from build123d import *

# Parameters (mm, degrees)
SKETCH1_W               = 110
SKETCH1_H               = 31.4
BOSS_EXTRUDE1_DEPTH     = 6
SKETCH2_R               = 2.54
SKETCH2_R_2             = 5
SKETCH2_R_3             = 2.5
CUT_EXTRUDE1_DEPTH      = 1
CUT_EXTRUDE1_DEPTH_BACK = 7


with BuildPart() as part:
    # Sketch1 → Boss-Extrude1 (new body)
    with BuildSketch(Plane(origin=(0, 0, 0), x_dir=(1, 0, 0), z_dir=(0, 1, 0))):
        Rectangle(SKETCH1_W, SKETCH1_H)
    extrude(amount=BOSS_EXTRUDE1_DEPTH)

    # Sketch2 → Cut-Extrude1 (cut, two sides)
    with BuildSketch(Plane(origin=(0, 6, 0), x_dir=(1, 0, 0), z_dir=(0, 1, 0))) as cut_extrude1_sk:
        with Locations((-10.4, 3)):
            Circle(SKETCH2_R)
        with Locations((-29.6, 3)):
            Circle(SKETCH2_R)
        with Locations((30, 0)):
            Circle(SKETCH2_R_2)
        with Locations((45, 0)):
            Circle(SKETCH2_R_3)
    extrude(amount=CUT_EXTRUDE1_DEPTH, mode=Mode.SUBTRACT)
    extrude(cut_extrude1_sk.sketch, amount=-CUT_EXTRUDE1_DEPTH_BACK, mode=Mode.SUBTRACT)


solid = part.part
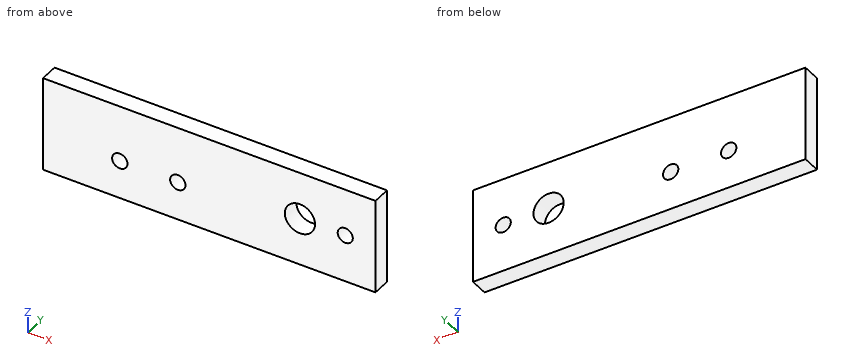
CAD build for the part. Positions are in the model's coordinates, mm. Round coordinates to 2 decimals unless told otherwise and drop trailing zeros. Write each loop counter-clockwise with the first axis right and the second up, starting at its lowest first coordinate (ties: lowest second). Pieces come first, ordered by that corner, then holes. Notation, with made-up numbers: M 57.25,80.5 L 73.25,80.5 A19 cw 73.25,101.5 Z; hole C 53,10.25 d1. An arc over 180 degrees is marked long. Put each result on its own line as item: value. Start each with the question number.
1) Saw through at A-A, the plane x = 30. Write the cut outline in (y, z).
2) Drill centre lines: probe 1 along X at (y, z) = (4.25, 0); probe 2 along Z at (x, y) = (-10.4, 1.5); probe 3 along X at (y, z) = (4.2, -3). Where is each one in solid material? Low to high. Write a range as [from, to].
3) Pin check, flat tip, straight feed: pin 1 Ø4.5 at (x, z) = (45, 0) entering from +Y. Stop position of the tip, or through.
4) Saw through at C-C, the plane y = 0.9. Write the cut outline in (x, z).
5) Saw through at D-D, the plane x = -29.6. Write the cut outline in (y, z).
6) Saw through at B-B, the plane z = 1.5. Write the cut outline in (x, y), and give its area (3 significant figures).
Resolved:
1. outline: M 0,-15.7 L 6,-15.7 L 6,-5 L 0,-5 Z; M 0,5 L 6,5 L 6,15.7 L 0,15.7 Z
2. probe 1: [-55, 25], [35, 42.5], [47.5, 55]
2. probe 2: [-15.7, -5.54], [-0.46, 15.7]
2. probe 3: [-55, -32.14], [-27.06, -12.94], [-7.86, 26], [34, 55]
3. pin 1: through
4. outline: M -55,-15.7 L 55,-15.7 L 55,15.7 L -55,15.7 Z; hole C -29.6,-3 d5.08; hole C -10.4,-3 d5.08; hole C 30,0 d10; hole C 45,0 d5
5. outline: M 0,-15.7 L 6,-15.7 L 6,-5.54 L 0,-5.54 Z; M 0,-0.46 L 6,-0.46 L 6,15.7 L 0,15.7 Z
6. outline: M -55,0 L 25.23,0 L 25.23,6 L -55,6 Z; M 34.77,0 L 43,0 L 43,6 L 34.77,6 Z; M 47,0 L 55,0 L 55,6 L 47,6 Z
6. area: 579 mm²
